```python
from build123d import *

# Parameters (mm, degrees)
PAD_DEPTH       = 20
CHAMFER_SIZE    = 1
CHAMFER001_SIZE = 2


with BuildPart() as part:
    # Sketch → Pad (new body)
    with BuildSketch(Plane.XY):
        Polygon((-7.5, 5), (-7.5, -8), (7.5, -8), (7.5, 5), (4.5, 5), (4.5, -5), (-4.5, -5), (-4.5, 5), align=None)
    extrude(amount=PAD_DEPTH)

    # Chamfer
    chamfer_edges = [part.edges().sort_by_distance(p)[0] for p in [
        (-4.5, 5, 10),
        (4.5, 5, 10),
    ]]
    chamfer(chamfer_edges, length=CHAMFER_SIZE)

    # Chamfer001
    chamfer001_edges = [part.edges().sort_by_distance(p)[0] for p in [
        (0, -8, 20),
        (0, -8, 0),
    ]]
    chamfer(chamfer001_edges, length=CHAMFER001_SIZE)


solid = part.part
```
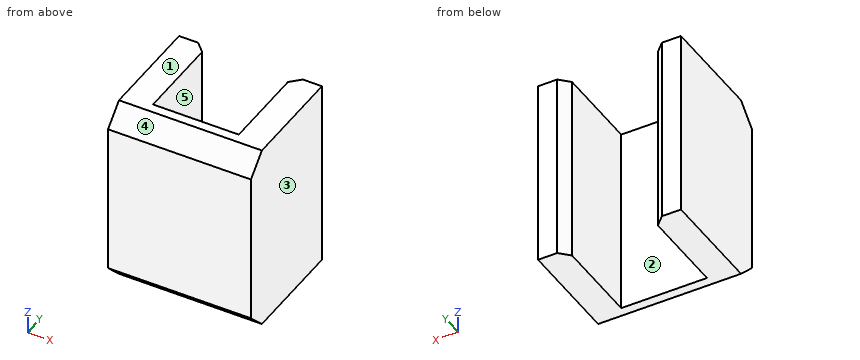
For this review, take the finished solid that the model builds, in its own axes (mm). Face numbers are marked on the shaded views. A direction names the side the tool comes from. Coordinates: 2 decimals unless noted, no trailing zeros. Loops run counter-clockwise (first coordinate to the right, second up) from the corner with the lowest first, then second, coordinate; pieces in that order, holes last.
1. For line 1 (X direction, y = 0.75, z = 15); line 2 (Y direction, x = 2.5, z = 14.25); line 3 (X direction, y = 4.75, z = 8), list the stretches that pass through material, from the lowest coordinate up.
2. Add section A-A, the plane y = -1. Give the boundary of the cut face in (x, z), then the cut area to 3 significant figures.
3. Mouldability with a two-part tool opening along X and no side actions: class the marked faces 3, 4 and 5 as +X half, -X half, draft (parallel to the pull), parting line (faces both ways), or undercut.
4. For the marked faces 1 and 2, list the 3-axis set-ups (+Z, -Z, +X, -X, +Y, -Y) from which the entire face can be reached by the end or side of a thin tool; tool diameter is ignored.
5. Add section B-B, the plane z = 6.25. Give the boundary of the cut face in (x, y).
6. Insertion check: P1, Ø6, axis at x = -2, z = 6.5, coming from the +Y side; P2, Ø4, axis at x = -2, z = 17.5, coming from the +Y side. Each pin has a flat end and moves straight along its axis. Give the tip position at first contact, or say it passes through.
7. Add section D-D, the plane z = 1.5. Give the boundary of the cut face in (x, y).
8. Add section C-C, the plane x = -6.5. Give the boundary of the cut face in (y, z).
Result:
1. line 1: x = -7.5 to -4.5, 4.5 to 7.5
1. line 2: y = -8 to -5
1. line 3: x = -7.5 to -5.25, 5.25 to 7.5
2. outline: (-7.5, 0) - (-4.5, 0) - (-4.5, 20) - (-7.5, 20) - close; (4.5, 0) - (7.5, 0) - (7.5, 20) - (4.5, 20) - close
2. area: 120 mm2
3. face 3: +X half
3. face 4: draft
3. face 5: undercut
4. face 1: +Z, +X, -X, +Y, -Y
4. face 2: +Z, -Z, +Y
5. outline: (-7.5, -8) - (7.5, -8) - (7.5, 5) - (5.5, 5) - (4.5, 4) - (4.5, -5) - (-4.5, -5) - (-4.5, 4) - (-5.5, 5) - (-7.5, 5) - close
6. P1: stops at y = 4.5
6. P2: stops at y = -5
7. outline: (-7.5, -7.5) - (7.5, -7.5) - (7.5, 5) - (5.5, 5) - (4.5, 4) - (4.5, -5) - (-4.5, -5) - (-4.5, 4) - (-5.5, 5) - (-7.5, 5) - close
8. outline: (-8, 2) - (-6, 0) - (5, 0) - (5, 20) - (-6, 20) - (-8, 18) - close
